Could you check a few things on this drawing? It's one solid part, dimensions in mm from its lowest x, y, z. A direction names the side the tool comes from. Round coordinates to 2 decimals unless told otherwise and drop trailing zeros. Write each loop counter-clockwise with the first axis right and the second up, starting at its lowest first coordinate (ties: lowest second). Pieces come first, ordered by that corner, then holes. Notation, with made-up numbers: (-10, -35) -> (17, -35) arc R21 ccw to (17, -7) -> close; hole circle Ø5 at (62.25, 78.25). An arc over 180 degrees is marked (long way). Return JSON: item names as keys, results as strings.
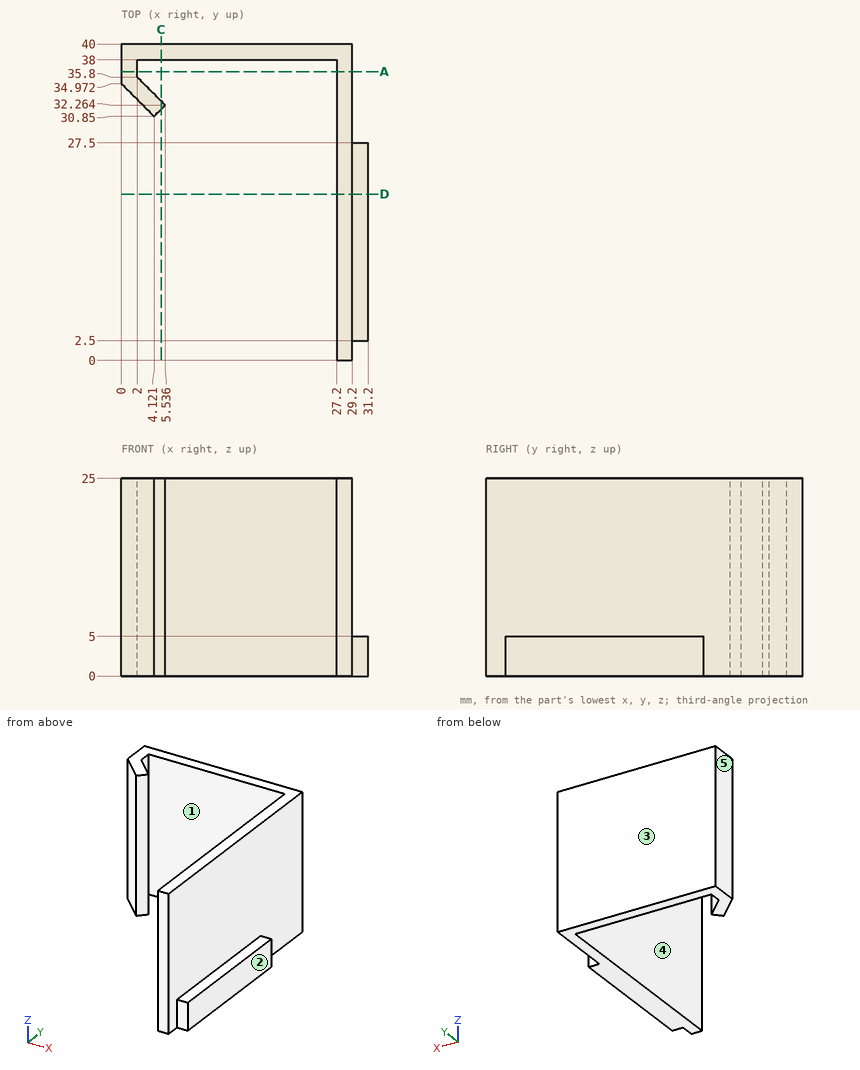
1) I want a section at A-A, the plane y = 36.5. Please give me the cut outline in (x, z), and give its area (3 significant figures).
Return value:
{"outline": "(0, 0) -> (2, 0) -> (2, 25) -> (0, 25) -> close; (27.2, 0) -> (29.2, 0) -> (29.2, 25) -> (27.2, 25) -> close", "area": "100 mm²"}
2) For the marked faces 4 and 5, which set-ups out of +Z, -Z, +X, -X, +Y, -Y let a thin tool reach every point of the face, with its end or its side?
Return value:
{"face 4": "+Z, -Z, -Y", "face 5": "+Z, -Z, -X, +Y, -Y"}
3) Thinking about a two-plate mould opening in X: for the marked faces 1, 2 and 3, which applies, pulls with the +X half, pulls with the -X half, needs draft (parallel to the pull), parting line crosses it, or undercut?
Return value:
{"face 1": "undercut", "face 2": "pulls with the +X half", "face 3": "needs draft"}
4) I want a section at C-C, the plane x = 5. Please give me the cut outline in (y, z).
Return value:
{"outline": "(31.73, 0) -> (32.8, 0) -> (32.8, 25) -> (31.73, 25) -> close; (38, 0) -> (40, 0) -> (40, 25) -> (38, 25) -> close"}
5) I want a section at D-D, the plane y = 21. Please give me the cut outline in (x, z).
Return value:
{"outline": "(27.2, 0) -> (31.2, 0) -> (31.2, 5) -> (29.2, 5) -> (29.2, 25) -> (27.2, 25) -> close"}
6) Will these pins go through, and if not, where does the flat tip stop? pin 1 Ø4 at (x, z) = (13, 6.5) entering from -Y; pin 2 Ø1.5 at (y, z) = (22, 12) entering from -X; pin 3 Ø0.6 at (x, y) = (30, 17.5) entering from +Z; pin 4 Ø10 at (x, y) = (22, 15) entering from -Z.
Return value:
{"pin 1": "y = 38", "pin 2": "x = 27.2", "pin 3": "z = 5", "pin 4": "through"}
7) If I drill on probe 1 along X at (y, z) = (17.5, 7.5); probe 2 along X at (y, z) = (21.5, 4.5); probe 3 along X at (y, z) = (35.5, 16.75), over which ranges is the centre line in solid material (lowest first)? Write a range as [from, to].
Return value:
{"probe 1": "[27.2, 29.2]", "probe 2": "[27.2, 31.2]", "probe 3": "[0, 2.3], [27.2, 29.2]"}
